```python
from build123d import *

# Parameters (mm, degrees)
SKETCH1_R           = 4.25
BOSS_EXTRUDE1_DEPTH = 20
SKETCH2_R           = 1.2
BOSS_EXTRUDE2_DEPTH = 0.8
SKETCH3_R           = 0.5
BOSS_EXTRUDE3_DEPTH = 5
SKETCH4_R           = 0.3
BOSS_EXTRUDE4_DEPTH = 1


with BuildPart() as part:
    # Sketch1 → Boss-Extrude1 (new body)
    with BuildSketch(Plane(origin=(0, 0, 0), x_dir=(0, 0, -1), z_dir=(1, 0, 0))):
        Circle(SKETCH1_R)
    extrude(amount=BOSS_EXTRUDE1_DEPTH)

    # Sketch2 → Boss-Extrude2 (add)
    with BuildSketch(Plane.ZY):
        Circle(SKETCH2_R)
    extrude(amount=BOSS_EXTRUDE2_DEPTH)

    # Sketch3 → Boss-Extrude3 (add)
    with BuildSketch(Plane.ZY.offset(0.8)):
        Circle(SKETCH3_R)
    extrude(amount=BOSS_EXTRUDE3_DEPTH)

    # Sketch4 → Boss-Extrude4 (add)
    with BuildSketch(Plane(origin=(20, 0, 0), x_dir=(0, 0, -1), z_dir=(1, 0, 0))):
        with Locations((-2.25, 0)):
            Circle(SKETCH4_R)
        with Locations((2.25, 0)):
            Circle(SKETCH4_R)
    extrude(amount=BOSS_EXTRUDE4_DEPTH)


solid = part.part
```
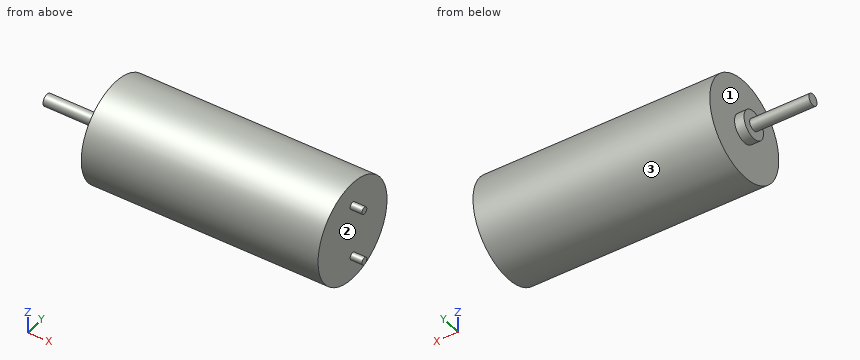
Part model, mm, in its own coordinate system. Face numbers are marked on the shaded views. Coordinates: 2 decimals unless noted, no trailing zeros. Order: outer loops, then holes, each group sorted by start corner. A loop starts at its lowest first (then second) coordinate and runs counter-clockwise, first axis right, second up. Notation, with made-up numbers: (34, 84.5) - (51, 84.5) arc R21 cw to (51, 99.5) - close; hole circle Ø2 at (36.25, 26.25). An arc over 180 degrees is marked (long way). Return JSON: item names as keys, results as strings. Group by question number.
Item 1: Cut at A-A (y = 0). List the corners of the cut face in (x, z), plus the area to 3 significant figures.
Item 2: Cut at D-D (z = 2.25). List the corners of the cut face in (x, y), plus the area to 3 significant figures.
Item 3: Cut at B-B (z = 0). List the corners of the cut face in (x, y).
Item 4: Drill centre lines: probe 1 along X at (y, z) = (2.5, 2); probe 2 along X at (y, z) = (-0.5, -1); probe 3 along Y at (x, z) = (8.5, -0.75). Where is each one in solid material? Low to high. Write a range as from..to.
Item 5: Pull direction X, two halves, no side cores. Call the marked faces 1, 2 and 3: pulls with the +X half, pulls with the -X half, needs draft (parallel to the pull), parting line crosses it, or undercut.
Item 6: Pin check, flat tips, straight feed: pin 1 (1.5 mm diameter, centred on x = 2, z = 2.5, fed in from +Y); pin 2 (4 mm diameter, centred on x = 17, z = 3, fed in from +Y); pin 3 (1 mm diameter, centred on y = 3, z = 0.5, fed in from +X). Stop position of each tip, or through.
Item 7: Cut at C-C (x = -2.5). List the corners of the cut face in (y, z).
Check values:
{
 "1": {"outline": "(-5.8, -0.5) - (-0.8, -0.5) - (-0.8, -1.2) - (0, -1.2) - (0, -4.25) - (20, -4.25) - (20, -2.55) - (21, -2.55) - (21, -1.95) - (20, -1.95) - (20, 1.95) - (21, 1.95) - (21, 2.55) - (20, 2.55) - (20, 4.25) - (0, 4.25) - (0, 1.2) - (-0.8, 1.2) - (-0.8, 0.5) - (-5.8, 0.5) - close", "area": "178 mm2"},
 "2": {"outline": "(0, -3.61) - (20, -3.61) - (20, -0.3) - (21, -0.3) - (21, 0.3) - (20, 0.3) - (20, 3.61) - (0, 3.61) - close", "area": "145 mm2"},
 "3": {"outline": "(-5.8, -0.5) - (-0.8, -0.5) - (-0.8, -1.2) - (0, -1.2) - (0, -4.25) - (20, -4.25) - (20, 4.25) - (0, 4.25) - (0, 1.2) - (-0.8, 1.2) - (-0.8, 0.5) - (-5.8, 0.5) - close"},
 "4": {"probe 1": "x = 0..20", "probe 2": "x = -0.8..20", "probe 3": "y = -4.18..4.18"},
 "5": {"face 1": "pulls with the -X half", "face 2": "pulls with the +X half", "face 3": "needs draft"},
 "6": {"pin 1": "stops at y = 3.87", "pin 2": "stops at y = 4.13", "pin 3": "stops at x = 20"},
 "7": {"outline": "circle Ø1 at (0, 0)"}
}
